Geometry: final body of the model. Coordinates: model frame, mm. A direction names the side the tool comes from. Coordinates: 2 decimals unless noted, no trailing zeros. Loops run counter-clockwise (first coordinate to the right, second up) from the corner with the lowest first, then second, coordinate; pieces in that order, holes last. Notation, with made-up numbers: (-5, 47) - (30, 47) arc R32 cw to (30, 83) - close; hole circle Ø3 at (11, -36.75). An arc over 180 degrees is marked (long way). Put each result on its own line as item: value. Start each with the question number.
1) Section A-A on y = 1.7. Output: boundary loops of the cut face in (x, z) (3 decimals).
2) Reachability of faces 1 (the flat face through (1, 0.94, -2)), 2 (the cylindrical face through (5.57, 0.15, -2.89)), 3 (the flat face through (2, 1.194, 1)) from +Z, -Z, +X, -X, +Y, -Y: full face, straight path, thin tool, end or side. Return the list, or none.
3) Draft query along X for faces 4 (the cylindrical face through (-2.846, 2.221, 0.374)), 5 (the flat face through (-3, 3.581, 0)), 6 (the cylindrical face through (3.18, 1.79, -1.65)), 7 (the cylindrical face through (1.93, 1.79, 2.52)). Return one class per face: +X half, -X half, draft (parallel to the pull), parting line (faces both ways), or undercut.
4) Material intervals for line 1 along X through (y, z) = (2.7, 0) (3 decimals); line 2 along Z through (x, y) = (-1, 2.6); line 3 along Y through (x, z) = (1.75, -4), sorted ascending. Write a range as from..to.
5) Contact query for flat-ended pins moving along their axis: pin 1 Ø2.5 at (x, z) = (1, 0) entering from -Y; pin 2 Ø6 at (x, z) = (3.5, -2.5) entering from -Y; pin 3 Ø1 at (y, z) = (1.5, 3.5) entering from +X. Output: stop coordinate, or through.
6) Section C-C on z = -4. Output: boundary loops of the cut face in (x, y).
7) Section B-B on x = 4.75. Output: boundary loops of the cut face in (y, z), and give its area (3 significant figures).
```python
from build123d import *

# Parameters (mm, degrees)
FILLET1_R = 0.254


with BuildPart() as part:
    # Sketch1 → Revolve1 (revolve)
    with BuildSketch(Plane.XY, mode=Mode.PRIVATE) as revolve1_sk:
        Polygon((-6.2738, 0), (-3.175, 0), (-3.175, 3.2766), (-2.8702, 3.2766), (-2.8702, 0.9398), (-1.4859, 0.9398), (-1.4859, 1.2446), (-1.7399, 1.2446), (-1.7399, 1.1938), (-2.413, 1.1938), (-2.413, 3.5814), (-3.5814, 3.5814), (-3.5814, 0.3048), (-6.2738, 0.3048), align=None)
    revolve(revolve1_sk.sketch.rotate(Axis((0, 0, 0), (0, 1, 0)), 270), axis=Axis((0, 0, 0), (0, 1, 0)))

    # Fillet1
    fillet1_edges = [part.edges().sort_by_distance(p)[0] for p in [
        (0, 0.9398, 2.8702),
        (0, 0.9398, 1.4859),
        (0, 3.5814, 2.413),
        (0, 3.5814, 3.5814),
        (0, 0, 3.175),
    ]]
    fillet(fillet1_edges, radius=FILLET1_R)


solid = part.part
```
Answer block:
1. outline: circle Ø7.163 at (0, 0); circle Ø5.74 at (0, 0); hole circle Ø6.35 at (0, 0); hole circle Ø4.826 at (0, 0)
2. face 1: -Y
2. face 2: +Y, -Y
2. face 3: +Y
3. face 4: undercut
3. face 5: draft
3. face 6: parting line
3. face 7: undercut
4. line 1: x = -3.581..-3.175, -2.87..-2.413, 2.413..2.87, 3.175..3.581
4. line 2: z = -3.44..-3.01, -2.69..-2.2, 2.2..2.69, 3.01..3.44
4. line 3: y = 0..0.3
5. pin 1: stops at y = 0.94
5. pin 2: stops at y = 0
5. pin 3: stops at x = 1.96
6. outline: (-4.83, 0) - (4.83, 0) - (4.83, 0.3) - (-4.83, 0.3) - close
7. outline: (0, -4.1) - (0.3, -4.1) - (0.3, 4.1) - (0, 4.1) - close
7. area: 2.50 mm²
